Check sheet for the drawn part. Datum: minimum x, y, z corner. Units: mm. A direction names the side the tool comes from. Coordinates: 2 decimals unless noted, no trailing zeros. Write each loop counter-clockwise with the first axis right and the second up, starting at its lowest first coordinate (ties: lowest second). Pieces come first, ordered by that corner, then holes. Notation, with made-up numbers: (9.5, -5.75) -> (37.5, -5.75) arc R25 ccw to (37.5, 20.25) -> close; hole circle Ø2 at (86.25, -34.5). An arc over 180 degrees is marked (long way). Answer in a Markdown table with one row per item. Add a question column.
1. Depth check by flat-ended pin: P1, Ø4, axis at x = 4.5, z = 11, coming from the +Y side; P2, Ø5, axis at x = 7.94, y = 7.94, coming from the +Z side. Enter the tip coordinate at first touch or a pass-through.
2. Cross-section at A-A on z = 21. Record the cut outline in (x, y) (1 decimal).
3. Cross-section at B-B on z = 44.5. Record the cut outline in (x, y) (1 decimal), and give its area (3 significant figures).
4. Mould release check, pull along X, two halves, no side actions. Record for the marked faces 1, 2 and 3: pulls with the +X half, pulls with the -X half, needs draft (parallel to the pull), parting line crosses it, or undercut.
5. Scan lines: L1, parallel to Z at x = 4.25, y = 2.5; L2, parallel to X at y = 6.75, z = 15.5 (1 decimal); L3, parallel to Y at x = 7.5, z = 22 (1 decimal). Record each from-to range of solid material in increasing order. Write a range as from..to.
6. Set-up check for the marked faces 4 and 5: record each of +Z, -Z, +X, -X, +Y, -Y from which the full face is reachable in a straight line by a thin tool's end or side.
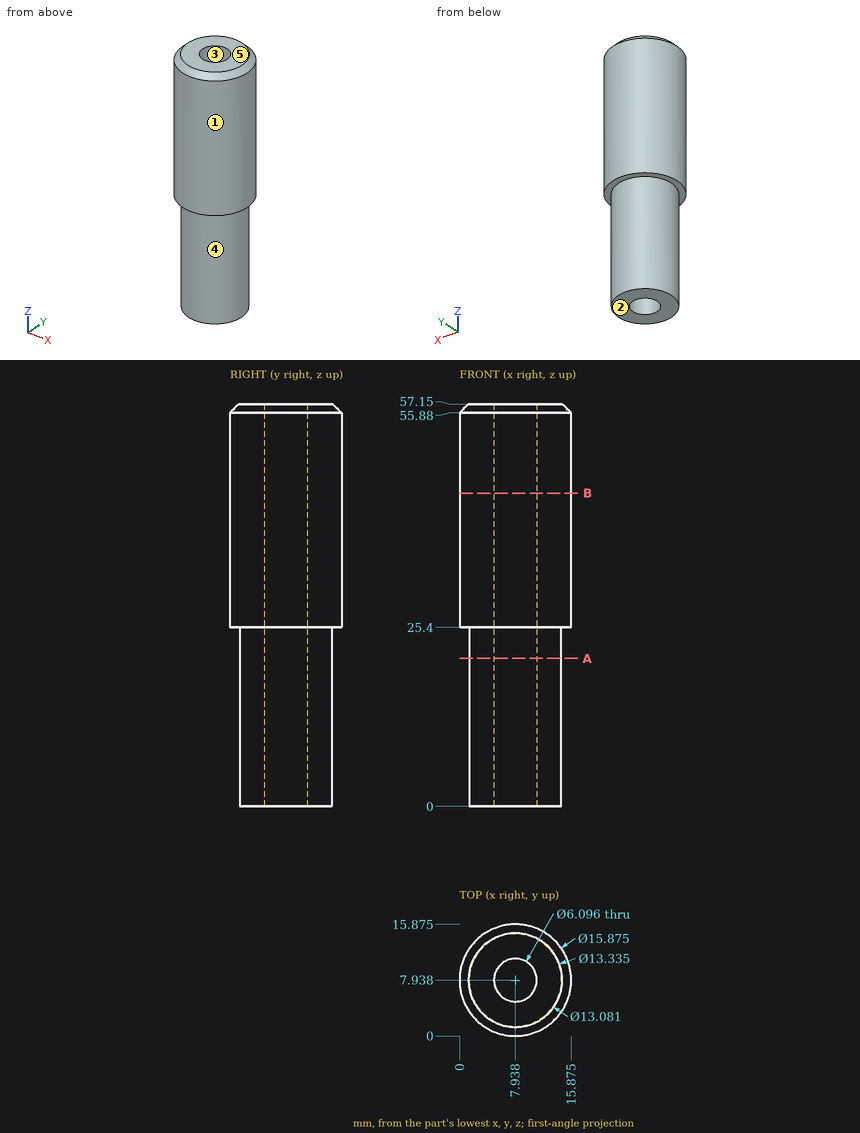
Results found:
| question | item | result |
|---|---|---|
| 1 | P1 | stops at y = 14.32 |
| 1 | P2 | passes through |
| 2 | outline | circle Ø13.1 at (7.9, 7.9); hole circle Ø6.1 at (7.9, 7.9) |
| 3 | outline | circle Ø15.9 at (7.9, 7.9); hole circle Ø6.1 at (7.9, 7.9) |
| 3 | area | 169 mm^2 |
| 4 | face 1 | parting line crosses it |
| 4 | face 2 | needs draft |
| 4 | face 3 | undercut |
| 5 | L1 | z = 25.4..57.15 |
| 5 | L2 | x = 1.5..5.1, 10.7..14.4 |
| 5 | L3 | y = 1.4..4.9, 11..14.5 |
| 6 | face 4 | -Z |
| 6 | face 5 | +Z, +X, -X, +Y, -Y |
